Input: dimensioned drawing with shaded views. Units: mm. Origin: part minimum x, y, z. A direction names the side the tool comes from. Give positions to 0.01 mm unless a question says otherwise; leave off trailing zeros. Order: outer loops, then holes, each group sorted by start corner. A loop starts at its lowest first (then second) coordinate and runs counter-clockwise, first axis right, second up. Notation, with made-up numbers: (14, -17) - (57, -17) arc R18 ccw to (57, 0) - close; hole circle Ø4 at (21.5, 64.5). An arc over 180 degrees is marked (long way). Use a Markdown table: item, result.
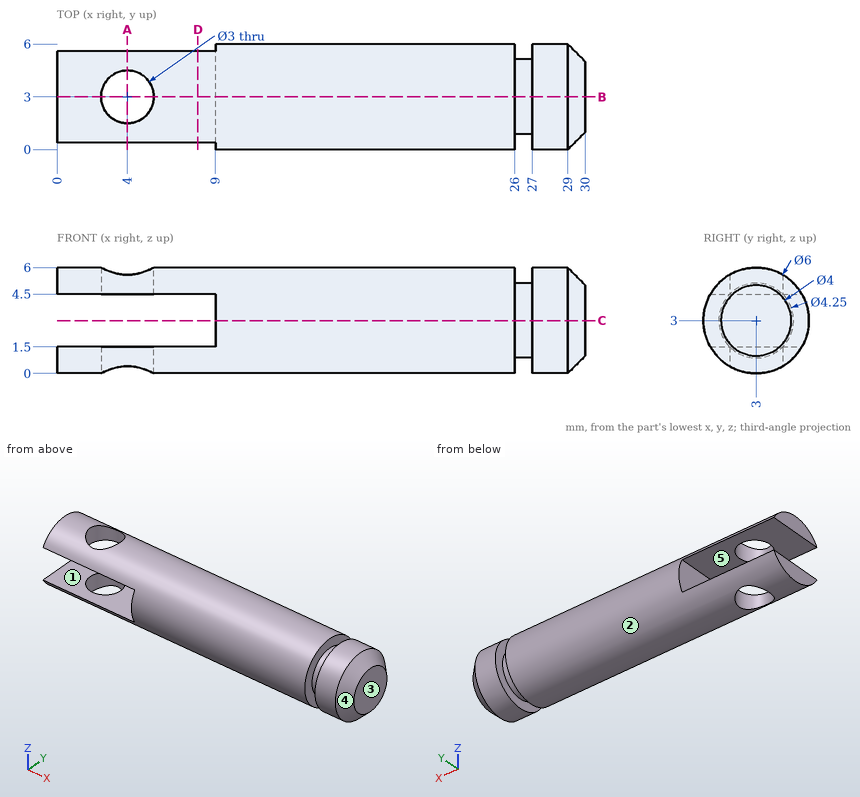
1. Section query B-B (y = 3). Return loops of the section in (x, z) (3 decimals).
Response:
| item | result |
|---|---|
| outline | (0, 0) - (2.5, 0) - (2.5, 1.5) - (0, 1.5) - close; (0, 4.5) - (2.5, 4.5) - (2.5, 6) - (0, 6) - close; (5.5, 0) - (26, 0) - (26, 0.875) - (27, 0.875) - (27, 0) - (29, 0) - (30, 1) - (30, 5) - (29, 6) - (27, 6) - (27, 5.125) - (26, 5.125) - (26, 6) - (5.5, 6) - (5.5, 4.5) - (9, 4.5) - (9, 1.5) - (5.5, 1.5) - close |
2. Material intervals for line 1 along Y through (x, z) = (4, 4.8); line 2 along X through (y, z) = (0.75, 1.75); line 3 along Z through (x, y) = (22.5, 4.5), sorted ascending.
Response:
| item | result |
|---|---|
| line 1 | y = 0.6 to 1.5, 4.5 to 5.4 |
| line 2 | x = 9 to 26, 27 to 29.43 |
| line 3 | z = 0.4 to 5.6 |
3. Pin query (flat end, axial travel): pin 1 (2 mm diameter, centred on x = 6, z = 2, fed in from +Y); pin 2 (1 mm diameter, centred on y = 3.5, z = 0.5, fed in from +X); pin 3 (1.5 mm diameter, centred on y = 3, z = 2.5, fed in from -X); pin 4 (2.5 mm diameter, centred on x = 4, y = 3, fed in from +Z). Return the tip coordinate at first contact, or that it passes through.
Response:
| item | result |
|---|---|
| pin 1 | stops at y = 5.6 |
| pin 2 | stops at x = 29.95 |
| pin 3 | stops at x = 9 |
| pin 4 | passes through |
4. Section query A-A (x = 4). Return loops of the section in (y, z).
Response:
| item | result |
|---|---|
| outline | (0.4, 1.5) arc R3 ccw to (1.5, 0.4) - (1.5, 1.5) - close; (0.4, 4.5) - (1.5, 4.5) - (1.5, 5.6) arc R3 ccw to start; (4.5, 0.4) arc R3 ccw to (5.6, 1.5) - (4.5, 1.5) - close; (4.5, 4.5) - (5.6, 4.5) arc R3 ccw to (4.5, 5.6) - close |
5. Set-up query: the marked faces 4 and 5. Return all of +Z, -Z, +X, -X, +Y, -Y with unobstructed straight access to the full face (end or side cutting, diameter ignored); none if empty.
Response:
| item | result |
|---|---|
| face 4 | +X |
| face 5 | -X, +Y, -Y |
6. Mould query, pull axis Z, two halves, no side actions, for the marked faces 1, 2 and 3. Classes: pulls with the +Z half, pulls with the -Z half, needs draft (parallel to the pull), parting line crosses it, or undercut.
Response:
| item | result |
|---|---|
| face 1 | undercut |
| face 2 | parting line crosses it |
| face 3 | needs draft |
7. Section query D-D (x = 8). Return loops of the section in (y, z).
Response:
| item | result |
|---|---|
| outline | (0.4, 1.5) arc R3 ccw to (5.6, 1.5) - close; (0.4, 4.5) - (5.6, 4.5) arc R3 ccw to start |
8. Section query C-C (z = 3). Return loops of the section in (x, y) (3 decimals).
Response:
| item | result |
|---|---|
| outline | (9, 0) - (26, 0) - (26, 0.875) - (27, 0.875) - (27, 0) - (29, 0) - (30, 1) - (30, 5) - (29, 6) - (27, 6) - (27, 5.125) - (26, 5.125) - (26, 6) - (9, 6) - close |
